from build123d import *

# Parameters (mm, degrees)
MODEL_R             = 13
MODEL_R_2           = 5.1
MODEL_R_3           = 10
MODEL_R_4           = 20
MODEL_R_5           = 29
MODEL_R_6           = 1.6
MODEL_R_7           = 2.1
BOSS_EXTRUDE1_DEPTH = 3
CUT_EXTRUDE1_REACH  = 162.618
SKETCH1_R           = 1.6


with BuildPart() as part:
    # Model → Boss-Extrude1 (new body)
    with BuildSketch(Plane.XY):
        with BuildLine():
            Line((-44.9, -110), (0, -110))
            Line((0, -110), (44.9, -110))
            ThreePointArc((44.9, -110), (50.059264201, -108.902545418), (54.325169295, -105.800212848))
            Line((54.325169295, -105.800212848), (106.229152519, -48.084515893))
            ThreePointArc((106.229152519, -48.084515893), (115.069026633, -32.588610118), (116.679519982, -14.821427412))
            Line((116.679519982, -14.821427412), (104.771085702, 81.023096559))
            ThreePointArc((104.771085702, 81.023096559), (82.034748438, 106.48766041), (50.189310486, 94.189159448))
            ThreePointArc((50.189310486, 94.189159448), (48.393618278, 92.581052005), (46.054195567, 92))
            Line((46.054195567, 92), (0, 92))
            Line((0, 92), (-46.054195567, 92))
            ThreePointArc((-46.054195567, 92), (-48.393618278, 92.581052005), (-50.189310486, 94.189159448))
            ThreePointArc((-50.189310486, 94.189159448), (-82.034748438, 106.48766041), (-104.771085702, 81.023096559))
            Line((-104.771085702, 81.023096559), (-116.679519982, -14.821427412))
            ThreePointArc((-116.679519982, -14.821427412), (-115.069026633, -32.588610118), (-106.229152519, -48.084515893))
            Line((-106.229152519, -48.084515893), (-54.325169295, -105.800212848))
            ThreePointArc((-54.325169295, -105.800212848), (-50.059264201, -108.902545418), (-44.9, -110))
        make_face()
        with Locations((0, -80)):
            Circle(MODEL_R, mode=Mode.SUBTRACT)
        with Locations((-44.9, -97.324116139)):
            Circle(MODEL_R_2, mode=Mode.SUBTRACT)
        with Locations((44.9, -97.324116139)):
            Circle(MODEL_R_2, mode=Mode.SUBTRACT)
        with Locations((0, 77.324116139)):
            Circle(MODEL_R_2, mode=Mode.SUBTRACT)
        Circle(MODEL_R_3, mode=Mode.SUBTRACT)
        with Locations((0, -40)):
            Circle(MODEL_R_3, mode=Mode.SUBTRACT)
        with Locations((0, 42.675883861)):
            Circle(MODEL_R_4, mode=Mode.SUBTRACT)
        with Locations((-37.5, 57.675883861)):
            Circle(MODEL_R_3, mode=Mode.SUBTRACT)
        with Locations((-37.5, 27.675883861)):
            Circle(MODEL_R_3, mode=Mode.SUBTRACT)
        with Locations((37.5, 57.675883861)):
            Circle(MODEL_R_3, mode=Mode.SUBTRACT)
        with Locations((37.5, 27.675883861)):
            Circle(MODEL_R_3, mode=Mode.SUBTRACT)
        with Locations((-75, -20)):
            Circle(MODEL_R_5, mode=Mode.SUBTRACT)
        with Locations((-75, 16.5)):
            Circle(MODEL_R_6, mode=Mode.SUBTRACT)
        with Locations((-100.809397513, 5.809397513)):
            Circle(MODEL_R_6, mode=Mode.SUBTRACT)
        with Locations((-49.190602487, 5.809397513)):
            Circle(MODEL_R_6, mode=Mode.SUBTRACT)
        with Locations((-38.5, -20)):
            Circle(MODEL_R_6, mode=Mode.SUBTRACT)
        with Locations((-49.190602487, -45.809397513)):
            Circle(MODEL_R_6, mode=Mode.SUBTRACT)
        with Locations((-75, -56.5)):
            Circle(MODEL_R_6, mode=Mode.SUBTRACT)
        with Locations((-100.809397513, -45.809397513)):
            Circle(MODEL_R_6, mode=Mode.SUBTRACT)
        with Locations((-111.5, -20)):
            Circle(MODEL_R_6, mode=Mode.SUBTRACT)
        with Locations((75, -20)):
            Circle(MODEL_R_5, mode=Mode.SUBTRACT)
        with Locations((75, 16.5)):
            Circle(MODEL_R_6, mode=Mode.SUBTRACT)
        with Locations((49.190602487, 5.809397513)):
            Circle(MODEL_R_6, mode=Mode.SUBTRACT)
        with Locations((100.809397513, 5.809397513)):
            Circle(MODEL_R_6, mode=Mode.SUBTRACT)
        with Locations((111.5, -20)):
            Circle(MODEL_R_6, mode=Mode.SUBTRACT)
        with Locations((100.809397513, -45.809397513)):
            Circle(MODEL_R_6, mode=Mode.SUBTRACT)
        with Locations((75, -56.5)):
            Circle(MODEL_R_6, mode=Mode.SUBTRACT)
        with Locations((49.190602487, -45.809397513)):
            Circle(MODEL_R_6, mode=Mode.SUBTRACT)
        with Locations((38.5, -20)):
            Circle(MODEL_R_6, mode=Mode.SUBTRACT)
        with Locations((-75, 77.324116139)):
            Circle(MODEL_R, mode=Mode.SUBTRACT)
        with Locations((75, 77.324116139)):
            Circle(MODEL_R, mode=Mode.SUBTRACT)
        with Locations((-75, 42.801273872)):
            Circle(MODEL_R, mode=Mode.SUBTRACT)
        with Locations((75, 42.675883861)):
            Circle(MODEL_R, mode=Mode.SUBTRACT)
        with Locations((-59.467622393, 92.856493746)):
            Circle(MODEL_R_7, mode=Mode.SUBTRACT)
        with Locations((-90.556349186, 92.880465325)):
            Circle(MODEL_R_7, mode=Mode.SUBTRACT)
        with Locations((-90.556349186, 61.767766953)):
            Circle(MODEL_R_7, mode=Mode.SUBTRACT)
        with Locations((-59.443650814, 61.767766953)):
            Circle(MODEL_R_7, mode=Mode.SUBTRACT)
        with Locations((90.532377607, 92.856493746)):
            Circle(MODEL_R_7, mode=Mode.SUBTRACT)
        with Locations((59.443650814, 92.880465325)):
            Circle(MODEL_R_7, mode=Mode.SUBTRACT)
        with Locations((59.443650814, 61.767766953)):
            Circle(MODEL_R_7, mode=Mode.SUBTRACT)
        with Locations((90.556349186, 61.767766953)):
            Circle(MODEL_R_7, mode=Mode.SUBTRACT)
        with Locations((15.532377607, -64.467622393)):
            Circle(MODEL_R_7, mode=Mode.SUBTRACT)
        with Locations((-15.556349186, -64.443650814)):
            Circle(MODEL_R_7, mode=Mode.SUBTRACT)
        with Locations((-15.556349186, -95.556349186)):
            Circle(MODEL_R_7, mode=Mode.SUBTRACT)
        with Locations((15.556349186, -95.556349186)):
            Circle(MODEL_R_7, mode=Mode.SUBTRACT)
        with BuildLine():
            Line((-37, 5), (-37, -5))
            ThreePointArc((-37, -5), (-34.9, -7.1), (-32.8, -5))
            Line((-32.8, -5), (-32.8, 5))
            ThreePointArc((-32.8, 5), (-34.9, 7.1), (-37, 5))
        make_face(mode=Mode.SUBTRACT)
        with BuildLine():
            Line((-37, -35), (-37, -45))
            ThreePointArc((-37, -45), (-34.9, -47.1), (-32.8, -45))
            Line((-32.8, -45), (-32.8, -35))
            ThreePointArc((-32.8, -35), (-34.9, -32.9), (-37, -35))
        make_face(mode=Mode.SUBTRACT)
        with BuildLine():
            Line((37, 5), (37, -5))
            ThreePointArc((37, -5), (34.9, -7.1), (32.8, -5))
            Line((32.8, -5), (32.8, 5))
            ThreePointArc((32.8, 5), (34.9, 7.1), (37, 5))
        make_face(mode=Mode.SUBTRACT)
        with BuildLine():
            Line((37, -35), (37, -45))
            ThreePointArc((37, -45), (34.9, -47.1), (32.8, -45))
            Line((32.8, -45), (32.8, -35))
            ThreePointArc((32.8, -35), (34.9, -32.9), (37, -35))
        make_face(mode=Mode.SUBTRACT)
        with BuildLine():
            Line((-62, -70), (-52, -70))
            ThreePointArc((-52, -70), (-49.9, -72.1), (-52, -74.2))
            Line((-52, -74.2), (-62, -74.2))
            ThreePointArc((-62, -74.2), (-64.1, -72.1), (-62, -70))
        make_face(mode=Mode.SUBTRACT)
        with BuildLine():
            Line((62, -70), (52, -70))
            ThreePointArc((52, -70), (49.9, -72.1), (52, -74.2))
            Line((52, -74.2), (62, -74.2))
            ThreePointArc((62, -74.2), (64.1, -72.1), (62, -70))
        make_face(mode=Mode.SUBTRACT)
    extrude(amount=BOSS_EXTRUDE1_DEPTH)

    # Sketch1 → Cut-Extrude1 (cut, up to next)
    with BuildSketch(Plane.XY.offset(3), mode=Mode.PRIVATE) as cut_extrude1_sk1:
        with Locations((-37.5, 42.675883861)):
            Circle(SKETCH1_R)
    cut_extrude1_tool1 = extrude(cut_extrude1_sk1.sketch, amount=-CUT_EXTRUDE1_REACH, mode=Mode.PRIVATE) & part.part
    # Sketch1 → Cut-Extrude1 (cut, up to next)
    with BuildSketch(Plane.XY.offset(3), mode=Mode.PRIVATE) as cut_extrude1_sk2:
        with Locations((37.5, 42.675883861)):
            Circle(SKETCH1_R)
    cut_extrude1_tool2 = extrude(cut_extrude1_sk2.sketch, amount=-CUT_EXTRUDE1_REACH, mode=Mode.PRIVATE) & part.part
    # Sketch1 → Cut-Extrude1 (cut, up to next)
    with BuildSketch(Plane.XY.offset(3), mode=Mode.PRIVATE) as cut_extrude1_sk3:
        with Locations((-20, -37.324116139)):
            Circle(SKETCH1_R)
    cut_extrude1_tool3 = extrude(cut_extrude1_sk3.sketch, amount=-CUT_EXTRUDE1_REACH, mode=Mode.PRIVATE) & part.part
    # Sketch1 → Cut-Extrude1 (cut, up to next)
    with BuildSketch(Plane.XY.offset(3), mode=Mode.PRIVATE) as cut_extrude1_sk4:
        with Locations((20, -37.324116139)):
            Circle(SKETCH1_R)
    cut_extrude1_tool4 = extrude(cut_extrude1_sk4.sketch, amount=-CUT_EXTRUDE1_REACH, mode=Mode.PRIVATE) & part.part
    add(cut_extrude1_tool1.solids().sort_by_distance((-37.5, 42.675884, 3))[0], mode=Mode.SUBTRACT)
    add(cut_extrude1_tool2.solids().sort_by_distance((37.5, 42.675884, 3))[0], mode=Mode.SUBTRACT)
    add(cut_extrude1_tool3.solids().sort_by_distance((-20, -37.324116, 3))[0], mode=Mode.SUBTRACT)
    add(cut_extrude1_tool4.solids().sort_by_distance((20, -37.324116, 3))[0], mode=Mode.SUBTRACT)


solid = part.part
Geometry: final body of the model. Coordinates: model frame, mm. Round coordinates to 2 decimals unless told otherwise and drop trailing zeros. Loops run counter-clockwise (first coordinate to the right, second up) from the corner with the lowest first, then second, coordinate; pieces in that order, holes last. Notation, with made-up numbers: M 59.5,8.5 L 116.5,8.5 A15 cw 116.5,28.5 Z; hole C 11,1.25 d2. An arc over 180 degrees is marked long. Put each result on its own line as item: value. Start each with the question number.
(1) Section query D-D (z = 1.85). State how many separate pieces and enclosed holes the cut face has, then the cut area to 3 significant figures.
(2) Section query A-A (y = 0). Return loops of the section in (x, z).
(3) Contact query for flat-ended pins moving along their axis: pin 1 Ø0.9 at (x, z) = (-1, 2) entering from +Y; pin 2 Ø4 at (x, y) = (51, -28) entering from +Z; pin 3 Ø0.9 at (y, z) = (-41, 1.5) entering from -X; pin 4 Ø0.9 at (y, z) = (0.5, 2) entering from -X. Output: stop coordinate, or through.
(4) Section query B-B (x = -96.5). Return loops of the section in (y, z).
(5) Material intervals for line 1 along X through (y, z) = (0.5, 1.3); line 2 along Y through (x, z) = (5.5, 1.3); line 3 along X through (y, z) = (68, 1.65), sorted ascending. Write a range as [from, to].
(6) Section query C-C (y = 86.5). Return loops of the section in (x, z), then the cut area to 3 significant figures.
(7) Draft query along Y for faces 1 (the face through (-28, 0, 3)), 2 (the face through (35.332, 47.914, 1.479)), 3 (the face through (-81.54, 106.603, 1.479)). Return one class per face: +Y half, -Y half, draft (parallel to the pull), parting line (faces both ways), or undercut.
Findings below:
1. separate pieces: 1
1. enclosed holes: 55
1. area: 29,900 mm2
2. outline: M -114.84,0 L -96,0 L -96,3 L -114.84,3 Z; M -54,0 L -37,0 L -37,3 L -54,3 Z; M -32.8,0 L -10,0 L -10,3 L -32.8,3 Z; M 10,0 L 32.8,0 L 32.8,3 L 10,3 Z; M 37,0 L 54,0 L 54,3 L 37,3 Z; M 96,0 L 114.84,0 L 114.84,3 L 96,3 Z
3. pin 1: stops at y = 92
3. pin 2: passes through
3. pin 3: stops at x = -111.63
3. pin 4: stops at x = -114.83
4. outline: M -58.9,0 L -39.46,0 L -39.46,3 L -58.9,3 Z; M -0.54,0 L 98.25,0 L 98.25,3 L -0.54,3 Z
5. line 1: x = [-114.78, -95.51], [-54.49, -37], [-32.8, -9.99], [9.99, 32.8], [37, 54.49], [95.51, 114.78]
5. line 2: y = [-110, -91.78], [-68.22, -48.35], [-31.65, -8.35], [8.35, 23.45], [61.9, 92]
5. line 3: x = [-106.39, -84.06], [-65.94, 65.94], [84.06, 106.39]
6. outline: M -103.56,0 L -84.21,0 L -84.21,3 L -103.56,3 Z; M -65.79,0 L 65.79,0 L 65.79,3 L -65.79,3 Z; M 84.21,0 L 103.56,0 L 103.56,3 L 84.21,3 Z
6. area: 511 mm2
7. face 1: draft
7. face 2: undercut
7. face 3: +Y half
